Geometry check sheet. Reference: the model listing, model coordinates, mm. A direction names the side the tool comes from. Give positions to 0.01 mm unless a question says otherwise; leave off trailing zeros. Loops run counter-clockwise (first coordinate to the right, second up) from the corner with the lowest first, then second, coordinate; pieces in that order, holes last.
```python
from build123d import *

# Parameters (mm, degrees)
PAD_DEPTH   = 55
FILLET_R    = 1
FILLET001_R = 1
FILLET002_R = 1
FILLET003_R = 1


with BuildPart() as part:
    # Sketch → Pad (new body)
    with BuildSketch(Plane.YZ):
        Polygon((0, 0), (63.157042, 0), (63.157042, 29.347581), (53.157042, 29.347581), (48.930859, 20.284503), (39.867781, 24.510686), (35.641599, 15.447608), (26.578521, 19.673791), (22.352338, 10.610713), (13.28926, 14.836895), (9.063078, 5.773817), (0, 10), align=None)
    extrude(amount=PAD_DEPTH)

    # Fillet
    fillet_edges = [part.edges().sort_by_distance(p)[0] for p in [
        (27.5, 13.28926, 14.836895),
        (27.5, 26.578521, 19.673791),
        (27.5, 39.867781, 24.510686),
        (27.5, 53.157042, 29.347581),
        (27.5, 0, 10),
    ]]
    fillet(fillet_edges, radius=FILLET_R)

    # Fillet001
    fillet001_edges = [part.edges().sort_by_distance(p)[0] for p in [
        (55, 18.273953, 12.512495),
        (55, 5.242848, 7.55522),
        (55, 31.563214, 17.34939),
        (55, 44.852474, 22.186285),
        (55, 50.909332, 24.527351),
    ]]
    fillet(fillet001_edges, radius=FILLET001_R)

    # Fillet002
    fillet002_edges = [part.edges().sort_by_distance(p)[0] for p in [
        (0, 44.852474, 22.186285),
        (0, 50.909332, 24.527351),
        (0, 31.563214, 17.34939),
        (0, 18.273953, 12.512495),
        (0, 5.242848, 7.55522),
    ]]
    fillet(fillet002_edges, radius=FILLET002_R)

    # Fillet003
    fillet003_edges = [part.edges().sort_by_distance(p)[0] for p in [
        (27.5, 63.157042, 29.347581),
        (0, 63.157042, 14.173791),
        (55, 63.157042, 14.173791),
    ]]
    fillet(fillet003_edges, radius=FILLET003_R)


solid = part.part
```
1) Depth check by flat-ended pin: P1, Ø12, axis at x = 49, z = 26.5, coming from the -Y side; P2, Ø5, axis at x = 45.5, z = 25, coming from the -Y side; P3, Ø2, axis at x = 42, z = 17.5, coming from the -Y side. Enter the tip coordinate at first touch or a pass-through.
2) Tool access check on faces 1 (the cylindrical face through (54.715, 50.94, 23.881)), 2 (the cylindrical face through (0.285, 37.575, 18.882)), 3 (the flat face through (27.129, 24.281, 14.746)). Record the directions out of +Z, -Z, +X, -X, +Y, -Y that give a thin tool (end or side, any length) a straight path to the whole face; none if there is none.
3) Mould release check, pull along Y, two halves, no side actions. Record for faces 4 (the flat face through (27, 0, 4)), 5 (the flat face through (55, 38, 11)), 6 (the cylindrical face through (0.285, 50.94, 23.881)), 7 (the flat face through (27.13, 44.91, 22.16)): +Y half, -Y half, draft (parallel to the pull), parting line (faces both ways), or undercut.
4) Sectioned sample at A-A on x = 41.5. Enter the section's corners in (y, z), plus the area to 3 significant figures.
5) Scan lines: line 1 along Y through (x, z) = (6, 13); line 2 along Y through (x, z) = (2.5, 6.75); line 3 along Y through (x, z) = (3.5, 25). Record each from-to range of solid material in increasing order.
Determined:
1. P1: stops at y = 38
1. P2: stops at y = 38.93
1. P3: stops at y = 25.1
2. face 1: +Z, +X
2. face 2: +Z, -X
2. face 3: +Z, +X, -X
3. face 4: -Y half
3. face 5: draft
3. face 6: undercut
3. face 7: undercut
4. outline: (0, 0) - (63.16, 0) - (63.16, 28.35) arc R1 ccw to (62.16, 29.35) - (53.79, 29.35) arc R1 ccw to (52.89, 28.77) - (48.93, 20.28) - (40.77, 24.09) arc R1 ccw to (39.45, 23.6) - (35.64, 15.45) - (27.48, 19.25) arc R1 ccw to (26.16, 18.77) - (22.35, 10.61) - (14.2, 14.41) arc R1 ccw to (12.87, 13.93) - (9.06, 5.77) - (1.42, 9.34) arc R1 ccw to (0, 8.43) - close
4. area: 1,140 mm2
5. line 1: y = 12.43 to 17.23, 23.47 to 63.16
5. line 2: y = 0 to 6.97, 9.52 to 63.16
5. line 3: y = 51.13 to 63.16
